```python
from build123d import *

# Parameters (mm, degrees)
SKETCH1_W           = 140
SKETCH1_H           = 80
BOSS_EXTRUDE1_DEPTH = 3
SKETCH2_W           = 100
SKETCH2_H           = 60
CUT_EXTRUDE1_DEPTH  = 13
SKETCH4_W           = 10
SKETCH4_H           = 3
BOSS_EXTRUDE2_DEPTH = 3


with BuildPart() as part:
    # Sketch1 → Boss-Extrude1 (new body)
    with BuildSketch(Plane(origin=(0, 0, 0), x_dir=(1, 0, 0), z_dir=(0, 1, 0))):
        Rectangle(SKETCH1_W, SKETCH1_H)
    extrude(amount=BOSS_EXTRUDE1_DEPTH)

    # Sketch2 → Cut-Extrude1 (cut)
    with BuildSketch(Plane(origin=(0, 3, 0), x_dir=(1, 0, 0), z_dir=(0, 1, 0))):
        with Locations((0, 10)):
            Rectangle(SKETCH2_W, SKETCH2_H)
    extrude(amount=-CUT_EXTRUDE1_DEPTH, mode=Mode.SUBTRACT)

    # Sketch4 → Boss-Extrude2 (add)
    with BuildSketch(Plane.XY.offset(40)):
        with Locations((-45, 1.5)):
            Rectangle(SKETCH4_W, SKETCH4_H)
        with Locations((-15, 1.5)):
            Rectangle(SKETCH4_W, SKETCH4_H)
        with Locations((15, 1.5)):
            Rectangle(SKETCH4_W, SKETCH4_H)
        with Locations((45, 1.5)):
            Rectangle(SKETCH4_W, SKETCH4_H)
    extrude(amount=BOSS_EXTRUDE2_DEPTH)


solid = part.part
```
Input: part model. Units: mm. Frame: model coordinates. A direction names the side the tool comes from. Give positions to 0.01 mm unless a question says otherwise; leave off trailing zeros. Order: outer loops, then holes, each group sorted by start corner. A loop starts at its lowest first (then second) coordinate and runs counter-clockwise, first axis right, second up.
1. Pin query (flat end, axial travel): pin 1 (1.5 mm diameter, centred on y = 1.5, z = 42, fed in from +X); pin 2 (1.5 mm diameter, centred on y = 2, z = 42, fed in from -X); pin 3 (1.5 mm diameter, centred on x = -32, y = 2, fed in from +Z). Return the tip coordinate at first contact, or that it passes through.
Derived:
pin 1: stops at x = 50
pin 2: stops at x = -50
pin 3: stops at z = 40
2. Reachability of faces 5 (the flat face through (-50, 2, -10)), 6 (the flat face through (-30, 1, 40)), 7 (the flat face through (-70, 1, 1)) from +Z, -Z, +X, -X, +Y, -Y: full face, straight path, thin tool, end or side. Return the list, or none.
Derived:
face 5: -Z, +Y, -Y
face 6: +Z, +Y, -Y
face 7: +Z, -Z, -X, +Y, -Y
3. Section A-A on z = -18.5. Return the cut outline in (x, y).
Derived:
outline: (-70, 0) - (-50, 0) - (-50, 3) - (-70, 3) - close; (50, 0) - (70, 0) - (70, 3) - (50, 3) - close
4. Section D-D on x = 11.5. Return the cut outline in (y, z), and give its area (3 significant figures).
Derived:
outline: (0, 20) - (3, 20) - (3, 43) - (0, 43) - close
area: 69.0 mm2
5. Material intervals for L1, parallel to X at y = 2.25, z = -1; L2, parallel to Z at x = -31, y = 1.35; L3, parallel to Z at x = -62.5, y = 2.65, sorted ascending.
Derived:
L1: x = -70 to -50, 50 to 70
L2: z = 20 to 40
L3: z = -40 to 40
6. Mould query, pull axis X, two halves, no side actions, for faces 1 (the flat face through (70, 1, 1)), 2 (the flat face through (-50, 1, 41)), 3 (the flat face through (20, 1, 41)), 4 (the flat face through (45, 2, 43)). Classes: released by +X, released by -X, zero draft, split by the parting line, or undercut.
Derived:
face 1: released by +X
face 2: released by -X
face 3: undercut
face 4: zero draft
7. Section C-C on x = -7. Return the cut outline in (y, z), and give its area (3 significant figures).
Derived:
outline: (0, 20) - (3, 20) - (3, 40) - (0, 40) - close
area: 60.0 mm2
8. Section B-B on y = 2.3. Return the cut outline in (x, z).
Derived:
outline: (-70, -40) - (-50, -40) - (-50, 20) - (50, 20) - (50, -40) - (70, -40) - (70, 40) - (50, 40) - (50, 43) - (40, 43) - (40, 40) - (20, 40) - (20, 43) - (10, 43) - (10, 40) - (-10, 40) - (-10, 43) - (-20, 43) - (-20, 40) - (-40, 40) - (-40, 43) - (-50, 43) - (-50, 40) - (-70, 40) - close
